Part model, mm, in its own coordinate system. A direction names the side the tool comes from. Give positions to 0.01 mm unless a question says otherwise; leave off trailing zeros. Write each loop counter-clockwise with the first axis right and the second up, starting at its lowest first coordinate (ties: lowest second). Pieces come first, ordered by that corner, then holes.
```python
from build123d import *

# Parameters (mm, degrees)
ESQUISSE1_W                 = 160
ESQUISSE1_H                 = 90
T_LE_DE_BASE_PLI_E1_DEPTH   = 3
T_LE_PLI_E_SUR_AR_TE1_DEPTH = 90
T_LE_PLI_E_SUR_AR_TE2_DEPTH = 90
EXTRUSION1_DEPTH            = 4
CONG_2_R                    = 1
CONG_3_R                    = 1
CONG_4_R                    = 1


# Sheet-metal steps are written as plain solids
with BuildPart() as part:
    # Esquisse1 → Tôle de base pliée1 (new body)
    with BuildSketch(Plane(origin=(0, 0, 0), x_dir=(1, 0, 0), z_dir=(0, 1, 0))):
        with Locations((-26.903987823, 16.826605784)):
            Rectangle(ESQUISSE1_W, ESQUISSE1_H)
    extrude(amount=T_LE_DE_BASE_PLI_E1_DEPTH)

    # Tôle pliée sur arête1 section (across the edge) → Tôle pliée sur arête1 (add)
    with BuildSketch(Plane(origin=(53.832612177, 0, -61.826605784), x_dir=(-1, 0, 0), z_dir=(0, 0, 1))):
        with BuildLine():
            Line((-3, 0.7366), (-3, 10))
            Line((-3, 10), (0, 10))
            Line((0, 10), (0, 0.7366))
            ThreePointArc((0, 0.7366), (0.215745145, 0.215745145), (0.7366, 0))
            Line((0.7366, 0), (0.7366, -3))
            ThreePointArc((0.7366, -3), (-1.905575199, -1.905575199), (-3, 0.7366))
        make_face()
    extrude(amount=T_LE_PLI_E_SUR_AR_TE1_DEPTH)

    # Tôle pliée sur arête2 section (across the edge) → Tôle pliée sur arête2 (add)
    with BuildSketch(Plane(origin=(-107.640587823, 0, 28.173394216), x_dir=(1, 0, 0), z_dir=(0, 0, -1))):
        with BuildLine():
            Line((-3, 0.7366), (-3, 10))
            Line((-3, 10), (0, 10))
            Line((0, 10), (0, 0.7366))
            ThreePointArc((0, 0.7366), (0.215745145, 0.215745145), (0.7366, 0))
            Line((0.7366, 0), (0.7366, -3))
            ThreePointArc((0.7366, -3), (-1.905575199, -1.905575199), (-3, 0.7366))
        make_face()
    extrude(amount=T_LE_PLI_E_SUR_AR_TE2_DEPTH)

    # Esquisse9 → Extrusion1 (add)
    with BuildSketch(Plane(origin=(0, 3, 0), x_dir=(1, 0, 0), z_dir=(0, 1, 0))):
        with BuildLine():
            Line((-100.504826498, 51.644704016), (-99.504826498, 51.644704016))
            Line((-99.504826498, 51.644704016), (-99.504826498, -18.355295984))
            Line((-99.504826498, -18.355295984), (-100.504826498, -18.355295984))
            ThreePointArc((-100.504826498, -18.355295984), (-102.626146841, -17.476616327), (-103.504826498, -15.355295984))
            Line((-103.504826498, -15.355295984), (-103.504826498, 48.644704016))
            ThreePointArc((-103.504826498, 48.644704016), (-102.626146841, 50.76602436), (-100.504826498, 51.644704016))
        make_face()
        with BuildLine():
            Line((45.696850851, 51.644704016), (45.696850851, -18.355295984))
            Line((45.696850851, -18.355295984), (46.696850851, -18.355295984))
            ThreePointArc((46.696850851, -18.355295984), (48.818171195, -17.476616327), (49.696850851, -15.355295984))
            Line((49.696850851, -15.355295984), (49.696850851, 48.644704016))
            ThreePointArc((49.696850851, 48.644704016), (48.818171195, 50.76602436), (46.696850851, 51.644704016))
            Line((46.696850851, 51.644704016), (45.696850851, 51.644704016))
        make_face()
    extrude(amount=EXTRUSION1_DEPTH)

    # Congé2
    cong_2_edges = [part.edges().sort_by_distance(p)[0] for p in [
        (-26.903987823, 3, -61.826605784),
        (55.738187375, 1.905575199, -61.826605784),
        (55.738187375, 1.905575199, 28.173394216),
        (53.616867032, -0.215745145, -61.826605784),
        (53.616867032, -0.215745145, 28.173394216),
        (53.832612177, -5.3683, 28.173394216),
        (53.832612177, -5.3683, -61.826605784),
        (56.832612177, -5.3683, 28.173394216),
        (56.832612177, -5.3683, -61.826605784),
        (-109.546163022, 1.905575199, 28.173394216),
        (-109.546163022, 1.905575199, -61.826605784),
        (-107.424842678, -0.215745145, 28.173394216),
        (-107.424842678, -0.215745145, -61.826605784),
        (-26.903987823, 0, -61.826605784),
        (-107.640587823, -5.3683, -61.826605784),
        (-107.640587823, -5.3683, 28.173394216),
        (-110.640587823, -5.3683, -61.826605784),
        (-110.640587823, -5.3683, 28.173394216),
        (-26.903987823, 0, 28.173394216),
        (-26.903987823, 3, 28.173394216),
    ]]
    fillet(cong_2_edges, radius=CONG_2_R)

    # Congé3
    cong_3_edges = [part.edges().sort_by_distance(p)[0] for p in [
        (-100.004826498, 7, -51.644704016),
        (-102.626146841, 7, -50.76602436),
        (-103.504826498, 7, -16.644704016),
        (-102.626146841, 7, 17.476616327),
        (-100.004826498, 7, 18.355295984),
        (48.818171195, 7, 17.476616327),
        (49.696850851, 7, -16.644704016),
        (48.818171195, 7, -50.76602436),
        (46.196850851, 7, -51.644704016),
        (46.196850851, 7, 18.355295984),
    ]]
    fillet(cong_3_edges, radius=CONG_3_R)

    # Congé4
    cong_4_edges = [part.edges().sort_by_distance(p)[0] for p in [
        (-100.004826498, 3, -51.644704016),
        (-102.626146841, 3, -50.76602436),
        (-103.504826498, 3, -16.644704016),
        (-102.626146841, 3, 17.476616327),
        (-100.004826498, 3, 18.355295984),
        (48.818171195, 3, 17.476616327),
        (49.696850851, 3, -16.644704016),
        (48.818171195, 3, -50.76602436),
        (46.196850851, 3, -51.644704016),
        (46.196850851, 3, 18.355295984),
    ]]
    fillet(cong_4_edges, radius=CONG_4_R)


solid = part.part
```
1) Saw through at C-C, the plane z = -29. Write the cut outline in (x, y).
Answers follow:
outline: (-110.64, -10) - (-107.64, -10) - (-107.64, -0.74) arc R0.74 cw to (-106.9, 0) - (53.1, 0) arc R0.74 cw to (53.83, -0.74) - (53.83, -10) - (56.83, -10) - (56.83, -0.74) arc R3.74 ccw to (53.1, 3) - (50.7, 3) arc R1 cw to (49.7, 4) - (49.7, 6) arc R1 ccw to (48.7, 7) - (45.7, 7) - (45.7, 3) - (-99.5, 3) - (-99.5, 7) - (-102.5, 7) arc R1 ccw to (-103.5, 6) - (-103.5, 4) arc R1 cw to (-104.5, 3) - (-106.9, 3) arc R3.74 ccw to (-110.64, -0.74) - close
2) 3-axis set-ups, long thin cutter, end or side, ignore diameter. For faces 1 (the face through (48.795, 4.986, 17.5)), 2 (the face through (53.833, -5, -17)), 3 (the face through (-99.505, 5, -17)): which of +Z, -Z, +X, -X, +Y, -Y reach the whole face in a straight line?
Answers follow:
face 1: +Z, +X, +Y
face 2: +Z, -Z, -Y
face 3: +Z, -Z, +Y
3) Saw through at A-A, the plane y = -2.75. Write the cut outline in (x, z), then the cut area to 3 significant figures.
Answers follow:
outline: (-110.64, -60.83) arc R1 ccw to (-109.64, -61.83) - (-108.64, -61.83) arc R1 ccw to (-107.64, -60.83) - (-107.64, 27.17) arc R1 ccw to (-108.64, 28.17) - (-109.64, 28.17) arc R1 ccw to (-110.64, 27.17) - close; (53.83, -60.83) arc R1 ccw to (54.83, -61.83) - (55.83, -61.83) arc R1 ccw to (56.83, -60.83) - (56.83, 27.17) arc R1 ccw to (55.83, 28.17) - (54.83, 28.17) arc R1 ccw to (53.83, 27.17) - close
area: 538 mm2
4) Pin check, flat tips, straight feed: pin 1 Ø4.5 at (y, z) = (4.5, -2) entering from -X; pin 2 Ø0.6 at (y, z) = (5, -1.5) entering from +X; pin 3 Ø1.6 at (y, z) = (5, -24) entering from -X; pin 4 Ø6 at (x, y) = (-27.5, -1) entering from +Z. Stop position of each tip, or through.
Answers follow:
pin 1: stops at x = -109.15
pin 2: stops at x = 49.7
pin 3: stops at x = -103.5
pin 4: stops at z = 28.17
5) Saw through at B-B, the plane x = -65. Write the cut outline in (y, z), then the cut area to 3 significant figures.
Answers follow:
outline: (0, -60.83) arc R1 ccw to (1, -61.83) - (2, -61.83) arc R1 ccw to (3, -60.83) - (3, 27.17) arc R1 ccw to (2, 28.17) - (1, 28.17) arc R1 ccw to (0, 27.17) - close
area: 269 mm2
6) Two-plate mould, pull along X, no slides. Class faces 4 (the face through (55.709, 1.934, -17.443)), 5 (the face through (-28, 3, -17)), 6 (the face through (-109, -10, -16)): +X half, -X half, draft (parallel to the pull), parting line (faces both ways), or undercut.
Answers follow:
face 4: +X half
face 5: undercut
face 6: draft
7) Saw through at D-D, the plane z = 22. Write the cut outline in (x, y), then the cut area to 3 significant figures.
Answers follow:
outline: (-110.64, -10) - (-107.64, -10) - (-107.64, -0.74) arc R0.74 cw to (-106.9, 0) - (53.1, 0) arc R0.74 cw to (53.83, -0.74) - (53.83, -10) - (56.83, -10) - (56.83, -0.74) arc R3.74 ccw to (53.1, 3) - (-106.9, 3) arc R3.74 ccw to (-110.64, -0.74) - close
area: 557 mm2
8) Wall check: L1, parallel to X at y = -5.5, z = -45; L2, parallel to X at y = 4, z = 10; L3, parallel to Y at x = 8, z = -22.5. Give the ranges that are in metal, low to high.
Answers follow:
L1: x = -110.64 to -107.64, 53.83 to 56.83
L2: x = -103.5 to -99.5, 45.7 to 49.7
L3: y = 0 to 3
